For this review, use the dimensioned drawing (mm, ordinates from the lowest corner) and the shaded views. Give positions to 0.01 mm unless a question says otherwise; leave off trailing zeros. Write each loop counter-clockwise with the first axis right and the second up, starting at its lowest first coordinate (ties: lowest second). Pieces come first, ordered by that corner, then holes. Notation, with made-up numbers: (65.25, 81.5) - (119.25, 81.5) arc R27 ccw to (119.25, 107.5) - close; hole circle Ø11 at (-17, -35). An arc over 180 degrees is marked (long way). One line per question, with ' | ' between items. Start each with the question number.
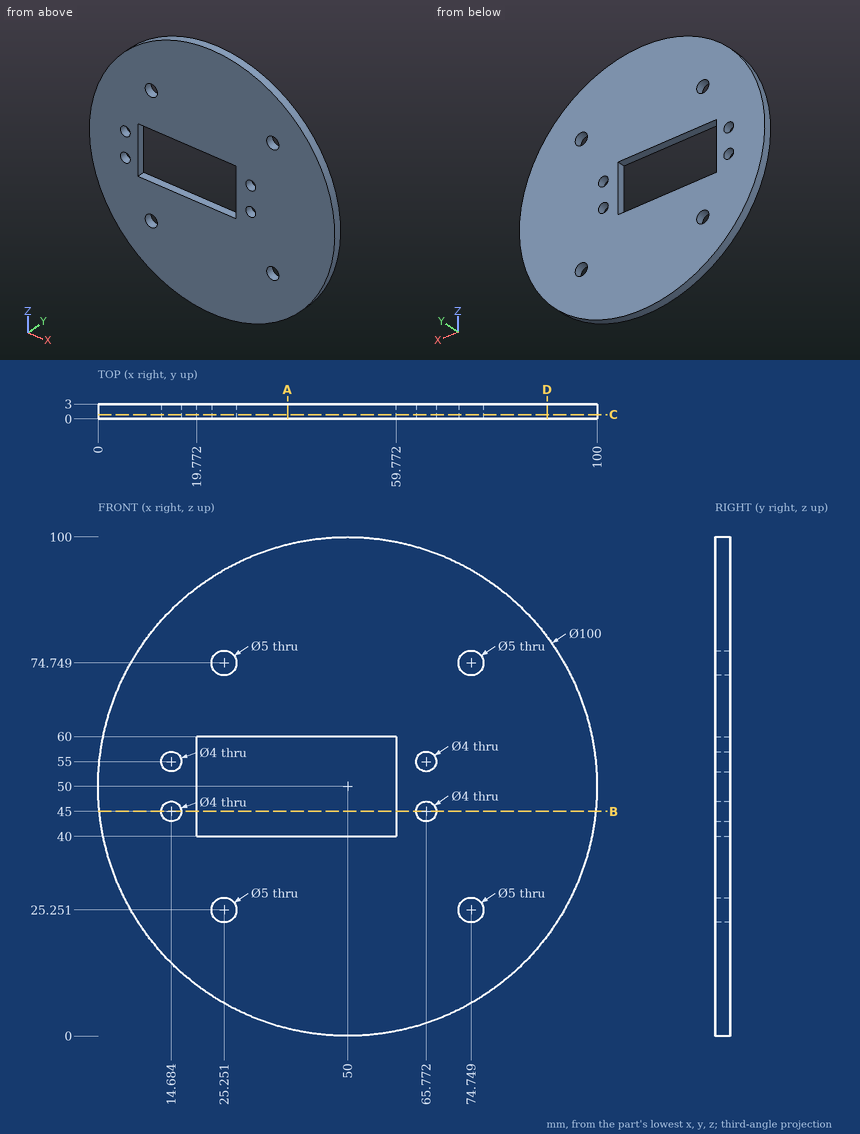
Item 1: Take a section at A-A (x = 38). Give the boundary of the cut face in (y, z), plus the area to 3 significant figures.
Item 2: Clearance check with flat-ended pins moving along their axes: P1, Ø1.5, axis at y = 2, z = 51.5, coming from the -X side; P2, Ø4, axis at x = 25.25, z = 74.75, coming from the -Y side; P3, Ø1, axis at x = 19, y = 0.5, coming from the -Z side; P4, Ø1, axis at y = 1, z = 47, coming from the -X side. State where each tip first meets the part, or that it passes through.
Item 3: For probe 1 along X at (y, z) = (1.15, 74.5); probe 2 along X at (y, z) = (1.85, 74) (1 decimal); probe 3 along X at (y, z) = (2, 48.5), list the stretches that pass through material, from the lowest coordinate up.
Item 4: Take a section at D-D (x = 90). Give the boundary of the cut face in (y, z).
Item 5: Take a section at C-C (y = 0.85). State how many separate pieces and enclosed holes the cut face has, plus the area to 4 significant figures.
Item 6: Take a section at B-B (z = 45). Give the boundary of the cut face in (x, y).
Check sheet entries:
1) outline: (0, 1.46) - (3, 1.46) - (3, 40) - (0, 40) - close; (0, 60) - (3, 60) - (3, 98.54) - (0, 98.54) - close | area: 231 mm^2
2) P1: stops at x = 0.01 | P2: passes through | P3: stops at z = 10.38 | P4: stops at x = 0.06
3) probe 1: x = 6.41 to 22.76, 27.74 to 72.26, 77.24 to 93.59 | probe 2: x = 6.1 to 22.9, 27.6 to 72.4, 77.1 to 93.9 | probe 3: x = 0.02 to 19.77, 59.77 to 99.98
4) outline: (0, 20) - (3, 20) - (3, 80) - (0, 80) - close
5) separate pieces: 1 | enclosed holes: 9 | area: 6,925 mm^2
6) outline: (0.25, 0) - (12.68, 0) - (12.68, 3) - (0.25, 3) - close; (16.68, 0) - (19.77, 0) - (19.77, 3) - (16.68, 3) - close; (59.77, 0) - (63.77, 0) - (63.77, 3) - (59.77, 3) - close; (67.77, 0) - (99.75, 0) - (99.75, 3) - (67.77, 3) - close
